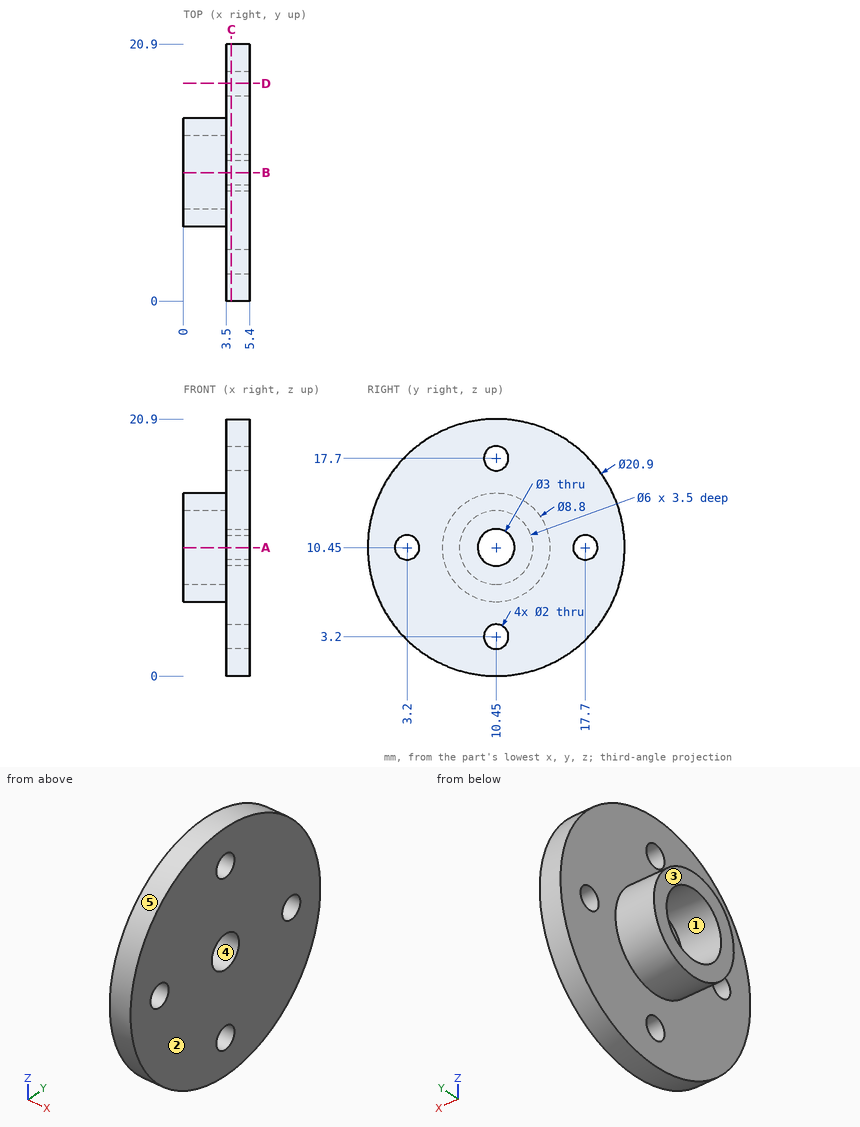
Design review of the part shown in the three views and the two pictorial views. Dimensions are in mm from the part's minimum x, y and z. A direction names the side the tool comes from. Give positions to 0.01 mm unless a question says otherwise; leave off trailing zeros. Loops run counter-clockwise (first coordinate to the right, second up) from the corner with the lowest first, then second, coordinate; pieces in that order, holes last. Notation, with made-up numbers: (69, -27) -> (112, -27) arc R4 cw to (112, -23) -> close; hole circle Ø5 at (-37.75, 71). An arc over 180 degrees is marked (long way). One line per question, with ' | ' between items.
1) We need section D-D (y = 17.7). Write out the cut boundary in (x, z).
Resolved:
outline: (3.5, 2.92) -> (5.4, 2.92) -> (5.4, 9.45) -> (3.5, 9.45) -> close; (3.5, 11.45) -> (5.4, 11.45) -> (5.4, 17.98) -> (3.5, 17.98) -> close
2) For the marked faces 1 and 2, list the 3-axis set-ups (+Z, -Z, +X, -X, +Y, -Y) from which the entire face can be reached by the end or side of a thin tool; tool diameter is ignored.
Resolved:
face 1: -X | face 2: +Z, -Z, +X, +Y, -Y
3) To check wall thickness, follow probe 1 along Y at (x, z) = (4.6, 10.45); probe 2 along X at (y, z) = (7.25, 6.5); probe 3 along Y at (x, z) = (4.6, 3.2). State the ranges of each line that lie inside material, in increasing order.
Resolved:
probe 1: y = 0 to 2.2, 4.2 to 8.95, 11.95 to 16.7, 18.7 to 20.9 | probe 2: x = 3.5 to 5.4 | probe 3: y = 2.92 to 9.45, 11.45 to 17.98
4) Insertion check: pin 1 Ø1.6 at (y, z) = (10.45, 3.2) entering from -X; pin 2 Ø8 at (y, z) = (18.5, 18) entering from -X; pin 3 Ø2 at (x, z) = (0.5, 14.5) entering from -Y; pin 4 Ø1 at (x, z) = (4, 12) entering from -Y. Each pin has a flat end and moves straight along its axis. Give the tip position at first contact, or say it passes through.
Resolved:
pin 1: passes through | pin 2: stops at x = 3.5 | pin 3: stops at y = 7.28 | pin 4: stops at y = 0.05
5) The part is to be moulded in two halves that separate along Z. For the marked faces 3, 4 and 5, say which applies: +Z half, -Z half, draft (parallel to the pull), parting line (faces both ways), or undercut.
Resolved:
face 3: draft | face 4: undercut | face 5: parting line
6) We need section A-A (z = 10.45). Write out the cut boundary in (x, y), plus the area to 3 significant figures.
Resolved:
outline: (0, 6.05) -> (3.5, 6.05) -> (3.5, 4.2) -> (5.4, 4.2) -> (5.4, 8.95) -> (3.5, 8.95) -> (3.5, 7.45) -> (0, 7.45) -> close; (0, 13.45) -> (3.5, 13.45) -> (3.5, 11.95) -> (5.4, 11.95) -> (5.4, 16.7) -> (3.5, 16.7) -> (3.5, 14.85) -> (0, 14.85) -> close; (3.5, 0) -> (5.4, 0) -> (5.4, 2.2) -> (3.5, 2.2) -> close; (3.5, 18.7) -> (5.4, 18.7) -> (5.4, 20.9) -> (3.5, 20.9) -> close | area: 36.2 mm2
7) We need section C-C (x = 3.9). Write out the cut boundary in (y, z), plus the area to 3 significant figures.
Resolved:
outline: circle Ø20.9 at (10.45, 10.45); hole circle Ø2 at (3.2, 10.45); hole circle Ø3 at (10.45, 10.45); hole circle Ø2 at (10.45, 3.2); hole circle Ø2 at (10.45, 17.7); hole circle Ø2 at (17.7, 10.45) | area: 323 mm2
